from build123d import *

# Parameters (mm, degrees)
F8_W      = 60.2088514067
F8_H      = 41.021
F9_DEPTH  = 2.032
F6_R      = 2.3749
F7_R      = 2.3749
F10_DEPTH = 12.192
F3_R      = 1.4605
F5_R      = 1.4605
F11_DEPTH = 12.192
F13_DEPTH = 2.286


with BuildPart() as f9:
    # F8 (on Top) → F9 (new body)
    with BuildSketch(Plane.XY):
        Rectangle(F8_W, F8_H)
    extrude(amount=F9_DEPTH)

    # F6 (on face) + F7 (on face) → F10 (cut)
    with BuildSketch(Plane.XY):
        with Locations((-23.9141, -15.367)):
            Circle(F6_R)
    with BuildSketch(Plane.XY):
        with Locations((23.9141, 15.367)):
            Circle(F7_R)
    extrude(amount=F10_DEPTH, mode=Mode.SUBTRACT)

    # F3 (on face) + F5 (on face) → F11 (cut)
    with BuildSketch(Plane.XY):
        with Locations((-24.5581628517, 15.367)):
            Circle(F3_R)
    with BuildSketch(Plane.XY):
        with Locations((24.5581628517, -15.367)):
            Circle(F5_R)
    extrude(amount=F11_DEPTH, mode=Mode.SUBTRACT)

    # F12 (on Top) → F13 (cut)
    with BuildSketch(Plane.XY):
        Polygon((-11.6205, -9.0932), (-11.6205, 11.811), (-17.4625, 11.811), (-17.4625, 5.5245), (-18.9865, 5.5245), (-18.9865, -2.8067), (-17.3355, -2.8067), (-17.3355, -9.0932), align=None)
    extrude(amount=F13_DEPTH, mode=Mode.SUBTRACT)


solid = f9.part
Input: part model. Units: mm. Frame: model coordinates. A direction names the side the tool comes from. Coordinates: 2 decimals unless noted, no trailing zeros. Loops run counter-clockwise (first coordinate to the right, second up) from the corner with the lowest first, then second, coordinate; pieces in that order, holes last. Notation, with made-up numbers: (3, 16) -> (40, 16) arc R33 cw to (40, 55) -> close; hole circle Ø5 at (-30, -5.5). An arc over 180 degrees is marked (long way). One line per item, written item: value.
(1) Cut plane A-A (y = 8.5). Output: boundary loops of the cut face in (x, z), then the cut area to 3 significant figures.
Answer below:
outline: (-30.1, 0) -> (-17.46, 0) -> (-17.46, 2.03) -> (-30.1, 2.03) -> close; (-11.62, 0) -> (30.1, 0) -> (30.1, 2.03) -> (-11.62, 2.03) -> close
area: 110 mm2
(2) Cut plane D-D (x = 24.5). Output: boundary loops of the cut face in (y, z).
Answer below:
outline: (-20.51, 0) -> (-16.83, 0) -> (-16.83, 2.03) -> (-20.51, 2.03) -> close; (-13.91, 0) -> (13.07, 0) -> (13.07, 2.03) -> (-13.91, 2.03) -> close; (17.67, 0) -> (20.51, 0) -> (20.51, 2.03) -> (17.67, 2.03) -> close
(3) Cut plane B-B (x = -16). Output: boundary loops of the cut face in (y, z).
Answer below:
outline: (-20.51, 0) -> (-9.09, 0) -> (-9.09, 2.03) -> (-20.51, 2.03) -> close; (11.81, 0) -> (20.51, 0) -> (20.51, 2.03) -> (11.81, 2.03) -> close
(4) Pin query (flat end, axial travel): pin 1 Ø2.5 at (x, y) = (24.56, -15.37) entering from -Z. Return the tip coordinate at first contact, or that it passes through.
Answer below:
pin 1: passes through
(5) Cut plane C-C (z = 0.9). Output: boundary loops of the cut face in (x, y).
Answer below:
outline: (-30.1, -20.51) -> (30.1, -20.51) -> (30.1, 20.51) -> (-30.1, 20.51) -> close; hole circle Ø4.75 at (-23.91, -15.37); hole circle Ø2.92 at (-24.56, 15.37); hole (-18.99, -2.81) -> (-17.34, -2.81) -> (-17.34, -9.09) -> (-11.62, -9.09) -> (-11.62, 11.81) -> (-17.46, 11.81) -> (-17.46, 5.52) -> (-18.99, 5.52) -> close; hole circle Ø4.75 at (23.91, 15.37); hole circle Ø2.92 at (24.56, -15.37)
(6) Set-up query: faces 1 (the face through (-18, -2.807, 1)), 2 (the face through (0, 20.51, 1)). Return all of +Z, -Z, +X, -X, +Y, -Y with unobstructed straight access to the full face (end or side cutting, diameter ignored); none if empty.
Answer below:
face 1: +Z, -Z
face 2: +Z, -Z, +X, -X, +Y
(7) Ray query, line 1 along X through (y, z) = (15.5, 1.6); line 2 along X through (y, z) = (-4, 1.85); line 3 along Y through (x, z) = (-12, 0.65). Return the intervals inside material, ascending.
Answer below:
line 1: x = -30.1 to -26.01, -23.1 to 21.54, 26.29 to 30.1
line 2: x = -30.1 to -17.34, -11.62 to 30.1
line 3: y = -20.51 to -9.09, 11.81 to 20.51
(8) Draft query along X for faces 3 (the face through (25.907, -15.926, 1.002)), 4 (the face through (-30.104, 0, 1)), 5 (the face through (0, 0, 2.032)). Return one class per face: pulls with the +X half, pulls with the -X half, needs draft (parallel to the pull), parting line crosses it, or undercut.
Answer below:
face 3: undercut
face 4: pulls with the -X half
face 5: needs draft
